```python
from build123d import *

# Parameters (mm, degrees)
SKETCH2_W                = 80
SKETCH2_H                = 58
BOSS_EXTRUDE1_DEPTH      = 40
SKETCH4_R                = 7.5
CUT_EXTRUDE7_DEPTH       = 58
CUT_EXTRUDE7_DEPTH_BACK  = 58
SKETCH12_W               = 36.66060556
SKETCH12_H               = 30
SKETCH12_W_2             = 17.33939444
CUT_EXTRUDE10_DEPTH      = 58
SKETCH14_W               = 16
SKETCH14_H               = 6
CUT_EXTRUDE11_DEPTH      = 58
CUT_EXTRUDE11_DEPTH_BACK = 58
SKETCH17_R               = 7
CUT_EXTRUDE12_DEPTH      = 58
CUT_EXTRUDE12_DEPTH_BACK = 58
CUT_EXTRUDE14_DEPTH      = 58
CUT_EXTRUDE14_DEPTH_BACK = 58
SKETCH20_R               = 7.5
CUT_EXTRUDE15_DEPTH      = 12
CUT_EXTRUDE16_DEPTH      = 6
SKETCH23_R               = 7.5
CUT_EXTRUDE17_DEPTH      = 12
CUT_EXTRUDE18_DEPTH      = 6


with BuildPart() as part:
    # Sketch2 → Boss-Extrude1 (new body)
    with BuildSketch(Plane(origin=(0, 0, 0), x_dir=(1, 0, 0), z_dir=(0, 1, 0))):
        Rectangle(SKETCH2_W, SKETCH2_H)
    extrude(amount=BOSS_EXTRUDE1_DEPTH)

    # Sketch4 → Cut-Extrude7 (cut, two sides)
    with BuildSketch(Plane.XY) as cut_extrude7_sk:
        with BuildLine():
            Line((-40, 40), (-40, 24))
            ThreePointArc((-40, 24), (-23.33939444, 35.82575695), (-3.33939444, 40))
            Line((-3.33939444, 40), (-6, 40))
            Line((-6, 40), (-40, 40))
        make_face()
        Polygon((25, 40), (40, 31.339745962), (40, 40), align=None)
        with Locations((-6, 19)):
            Circle(SKETCH4_R)
        Polygon((25, 0), (40, 0), (40, 8.660254038), align=None)
    extrude(amount=CUT_EXTRUDE7_DEPTH, mode=Mode.SUBTRACT)
    extrude(cut_extrude7_sk.sketch, amount=-CUT_EXTRUDE7_DEPTH_BACK, mode=Mode.SUBTRACT)

    # Sketch12 → Cut-Extrude10 (cut)
    with BuildSketch(Plane(origin=(0, 40, 0), x_dir=(1, 0, 0), z_dir=(0, 1, 0))):
        with Locations((-21.66969722, 0)):
            Rectangle(SKETCH12_W, SKETCH12_H)
        with Locations((5.33030278, 0)):
            Rectangle(SKETCH12_W_2, SKETCH12_H)
    extrude(amount=-CUT_EXTRUDE10_DEPTH, mode=Mode.SUBTRACT)

    # Sketch14 → Cut-Extrude11 (cut, two sides)
    with BuildSketch(Plane(origin=(0, 40, 0), x_dir=(1, 0, 0), z_dir=(0, 1, 0))) as cut_extrude11_sk:
        with Locations((-32, 18)):
            Rectangle(SKETCH14_W, SKETCH14_H)
        with Locations((-32, -18)):
            Rectangle(SKETCH14_W, SKETCH14_H)
    extrude(amount=CUT_EXTRUDE11_DEPTH, mode=Mode.SUBTRACT)
    extrude(cut_extrude11_sk.sketch, amount=-CUT_EXTRUDE11_DEPTH_BACK, mode=Mode.SUBTRACT)

    # Sketch17 → Cut-Extrude12 (cut, two sides)
    with BuildSketch(Plane(origin=(40, 0, 0), x_dir=(0, 0, -1), z_dir=(1, 0, 0))) as cut_extrude12_sk:
        with Locations((0, 20)):
            Circle(SKETCH17_R)
    extrude(amount=CUT_EXTRUDE12_DEPTH, mode=Mode.SUBTRACT)
    extrude(cut_extrude12_sk.sketch, amount=-CUT_EXTRUDE12_DEPTH_BACK, mode=Mode.SUBTRACT)

    # Sketch19 → Cut-Extrude14 (cut, two sides)
    with BuildSketch(Plane(origin=(0, 40, 0), x_dir=(1, 0, 0), z_dir=(0, 1, 0))) as cut_extrude14_sk:
        Polygon((25, 29), (40, 29), (40, 14), align=None)
        Polygon((25, -29), (40, -14), (40, -29), align=None)
    extrude(amount=CUT_EXTRUDE14_DEPTH, mode=Mode.SUBTRACT)
    extrude(cut_extrude14_sk.sketch, amount=-CUT_EXTRUDE14_DEPTH_BACK, mode=Mode.SUBTRACT)

    # Sketch20 → Cut-Extrude15 (cut)
    with BuildSketch(Plane.XY.offset(29)):
        with BuildLine():
            Line((23, 2), (23, 38))
            Line((23, 38), (-4, 38))
            ThreePointArc((-4, 38), (-13.167101456, 37.028245592), (-22, 34.39007216))
            Line((-22, 34.39007216), (-22, 2))
            Line((-22, 2), (23, 2))
        make_face()
        with Locations((-6, 19)):
            Circle(SKETCH20_R, mode=Mode.SUBTRACT)
    extrude(amount=-CUT_EXTRUDE15_DEPTH, mode=Mode.SUBTRACT)

    # Sketch22 → Cut-Extrude16 (cut)
    with BuildSketch(Plane.XY.offset(29)):
        with BuildLine():
            Line((-22, 2), (-40, 2))
            Line((-40, 2), (-40, 22))
            ThreePointArc((-40, 22), (-31.685151748, 29.190408126), (-22, 34.39007216))
            Line((-22, 34.39007216), (-22, 2))
        make_face()
    extrude(amount=-CUT_EXTRUDE16_DEPTH, mode=Mode.SUBTRACT)

    # Sketch23 → Cut-Extrude17 (cut)
    with BuildSketch(Plane(origin=(0, 0, -29), x_dir=(-1, 0, 0), z_dir=(0, 0, -1))):
        with BuildLine():
            Line((4, 38), (-23, 38))
            Line((-23, 38), (-23, 2))
            Line((-23, 2), (22, 2))
            Line((22, 2), (22, 34.39007216))
            ThreePointArc((22, 34.39007216), (13.167101456, 37.028245592), (4, 38))
        make_face()
        with Locations((6, 19)):
            Circle(SKETCH23_R, mode=Mode.SUBTRACT)
    extrude(amount=-CUT_EXTRUDE17_DEPTH, mode=Mode.SUBTRACT)

    # Sketch24 → Cut-Extrude18 (cut)
    with BuildSketch(Plane(origin=(0, 0, -29), x_dir=(-1, 0, 0), z_dir=(0, 0, -1))):
        with BuildLine():
            Line((22, 2), (40, 2))
            Line((40, 2), (40, 22))
            ThreePointArc((40, 22), (31.685151748, 29.190408126), (22, 34.39007216))
            Line((22, 34.39007216), (22, 2))
        make_face()
    extrude(amount=-CUT_EXTRUDE18_DEPTH, mode=Mode.SUBTRACT)


solid = part.part
```
Source: CAD feature listing. Evaluate the final solid. Frame: model axes, mm. A direction names the side the tool comes from. Coordinates: 2 decimals unless noted, no trailing zeros. Write each loop counter-clockwise with the first axis right and the second up, starting at its lowest first coordinate (ties: lowest second). Pieces come first, ordered by that corner, then holes. Notation, with made-up numbers: (-15.75, -8) - (9.25, -8) arc R16 ccw to (9.25, 19) - close; hole circle Ø5 at (67, 43.25). An arc over 180 degrees is marked (long way). Answer as a JSON object with one key per item and string values.
Q1. Section query D-D, the plane y = 18. State how many separate pieces and enclosed holes the cut face has, plus the area to 3 significant figures.
Ans:
{"separate pieces": "4", "enclosed holes": "0", "area": "899 mm2"}
Q2. First-contact query: pin 1 Ø19.5 at (x, y) = (-6, 19) entering from -Z; pin 2 Ø3 at (y, z) = (10.5, 5.5) entering from -X; pin 3 Ø6.5 at (y, z) = (21.5, -20.5) entering from +X. Flat tips, straight axial feed; report the tip coordinate or a pass-through.
Ans:
{"pin 1": "stops at z = -17", "pin 2": "stops at x = 14", "pin 3": "stops at x = 36.75"}
Q3. Set-up query: faces 1 (the flat face through (10, 38, 23)), 2 (the flat face through (-1, 0, -20)), 3 (the flat face through (-24, 18, 18)), 4 (the flat face through (-22, 18, -20)). Return all of +Z, -Z, +X, -X, +Y, -Y with unobstructed straight access to the full face (end or side cutting, diameter ignored); none if empty.
Ans:
{"face 1": "+Z", "face 2": "+Z, -Z, +X, -X, -Y", "face 3": "-X, +Y, -Y", "face 4": "-Z"}
Q4. Section query B-B, the plane x = 19. Output: boundary loops of the cut face in (y, z).
Ans:
{"outline": "(0, -29) - (2, -29) - (2, -17) - (38, -17) - (38, -29) - (40, -29) - (40, 29) - (38, 29) - (38, 17) - (2, 17) - (2, 29) - (0, 29) - close; hole circle Ø14 at (20, 0)"}
Q5. Material intervals for line 1 (Z direction, x = -20.5, y = 14.5); line 2 (Z direction, x = -25.5, y = 13); line 3 (Y direction, x = 19, z = -25.5), sorted ascending. Write a range as [from, to].
Ans:
{"line 1": "z = [-17, -15], [15, 17]", "line 2": "z = [-23, -21], [21, 23]", "line 3": "y = [0, 2], [38, 40]"}
Q6. Section query A-A, the plane z = 0. Output: boundary loops of the cut face in (x, y), plus the area to 3 significant figures.
Ans:
{"outline": "(14, 0) - (25, 0) - (40, 8.66) - (40, 13) - (14, 13) - close; (14, 27) - (40, 27) - (40, 31.34) - (25, 40) - (14, 40) - close", "area": "546 mm2"}
Q7. Draft query along X for faces 5 (the flat face through (-1, 25, -15)), 6 (the flat face through (9, 38, -23)), 7 (the flat face through (33, 20, -21)). Return one class per face: released by +X, released by -X, zero draft, split by the parting line, or undercut.
Ans:
{"face 5": "zero draft", "face 6": "undercut", "face 7": "released by +X"}
Q8. Section query C-C, the plane x = 5. Output: boundary loops of the cut face in (y, z).
Ans:
{"outline": "(0, -29) - (2, -29) - (2, -17) - (38, -17) - (38, -29) - (40, -29) - (40, -15) - (0, -15) - close; (0, 15) - (40, 15) - (40, 29) - (38, 29) - (38, 17) - (2, 17) - (2, 29) - (0, 29) - close"}
